CAD build for the part. Positions are in the model's coordinates, mm. Face numbers are marked on the shaded views. A direction names the side the tool comes from. Give positions to 0.01 mm unless a question says otherwise; leave off trailing zeros. Order: outer loops, then holes, each group sorted by start corner. A loop starts at its lowest first (then second) coordinate and runs counter-clockwise, first axis right, second up. Notation, with made-up numbers: (29.25, -18.75) -> (58.25, -18.75) arc R33 ccw to (58.25, 17.25) -> close; hole circle Ø8 at (-24.75, -6). An arc over 180 degrees is marked (long way). Answer as CSV lines item,"result".
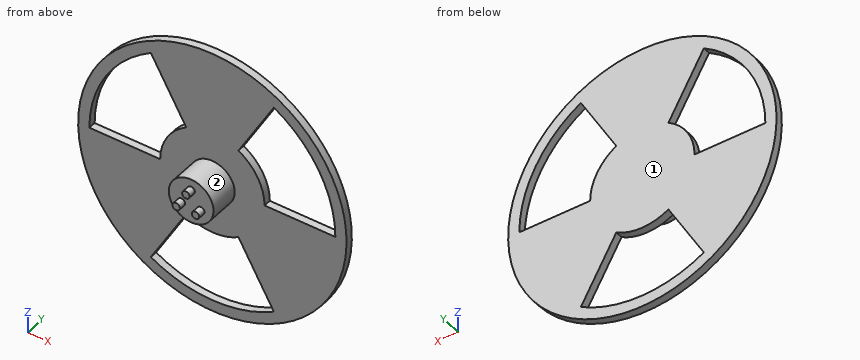
```python
from build123d import *

# Parameters (mm, degrees)
SKETCH1_R                = 18
BOSS_EXTRUDE1_DEPTH      = 1
SKETCH4_R                = 0.5
CUT_EXTRUDE2_DEPTH       = 1
BOSS_EXTRUDE2_DEPTH      = 4
BOSS_EXTRUDE2_DEPTH_BACK = 1
SKETCH5_R                = 3
BOSS_EXTRUDE3_START      = -5
SKETCH4_3_R              = 0.5
BOSS_EXTRUDE3_DEPTH      = 1


with BuildPart() as part:
    # Sketch1 → Boss-Extrude1 (new body)
    with BuildSketch(Plane(origin=(0, 0, 0), x_dir=(1, 0, 0), z_dir=(0, 1, 0))):
        with Locations(Location((0, 0, 0), (0, 0, 270))):
            Circle(SKETCH1_R)
    extrude(amount=BOSS_EXTRUDE1_DEPTH)

    # Sketch4 → Cut-Extrude2 (cut)
    with BuildSketch(Plane(origin=(0, 1, 0), x_dir=(1, 0, 0), z_dir=(0, 1, 0))):
        with Locations(Location((1.299038106, 0.75, 0), (0, 0, 270))):
            Circle(SKETCH4_R)
        with Locations(Location((0, -1.5, 0), (0, 0, 270))):
            Circle(SKETCH4_R)
        with Locations(Location((-1.299038106, 0.75, 0), (0, 0, 270))):
            Circle(SKETCH4_R)
        with BuildLine():
            Line((-3.5, 6.062177826), (-8.25, 14.289419162))
            ThreePointArc((-8.25, 14.289419162), (0, 16.5), (8.25, 14.289419162))
            Line((8.25, 14.289419162), (3.5, 6.062177826))
            ThreePointArc((3.5, 6.062177826), (0, 7), (-3.5, 6.062177826))
        make_face()
        with BuildLine():
            Line((7, 0), (16.5, 0))
            ThreePointArc((16.5, 0), (14.289419162, -8.25), (8.25, -14.289419162))
            Line((8.25, -14.289419162), (3.5, -6.062177826))
            ThreePointArc((3.5, -6.062177826), (6.062177826, -3.5), (7, 0))
        make_face()
        with BuildLine():
            Line((-3.5, -6.062177826), (-8.25, -14.289419162))
            ThreePointArc((-8.25, -14.289419162), (-14.289419162, -8.25), (-16.5, 0))
            Line((-16.5, 0), (-7, 0))
            ThreePointArc((-7, 0), (-6.062177826, -3.5), (-3.5, -6.062177826))
        make_face()
    extrude(amount=-CUT_EXTRUDE2_DEPTH, mode=Mode.SUBTRACT)

    # Sketch5 → Boss-Extrude2 (add, two sides: drawn at the far end of the back side and taken through both)
    with BuildSketch(Plane.XZ.offset(-BOSS_EXTRUDE2_DEPTH_BACK)):
        with Locations(Location((0, 0, 0), (0, 0, 270))):
            Circle(SKETCH5_R)
    extrude(amount=BOSS_EXTRUDE2_DEPTH + BOSS_EXTRUDE2_DEPTH_BACK)

    # Sketch4<3> → Boss-Extrude3 (add)
    with BuildSketch(Plane(origin=(0, 1, 0), x_dir=(1, 0, 0), z_dir=(0, 1, 0)).offset(BOSS_EXTRUDE3_START)):
        with Locations(Location((0, -1.5, 0), (0, 0, 90))):
            Circle(SKETCH4_3_R)
        with Locations(Location((-1.299038106, 0.75, 0), (0, 0, 90))):
            Circle(SKETCH4_3_R)
        with Locations(Location((1.299038106, 0.75, 0), (0, 0, 90))):
            Circle(SKETCH4_3_R)
    extrude(amount=-BOSS_EXTRUDE3_DEPTH)


solid = part.part
```
1) Band-saw the part on B-B, the plane z = 12.5. Write the cut outline in (x, y).
Data:
outline,"(-12.95, 0) -> (-10.77, 0) -> (-10.77, 1) -> (-12.95, 1) -> close; (-7.22, 0) -> (7.22, 0) -> (7.22, 1) -> (-7.22, 1) -> close; (10.77, 0) -> (12.95, 0) -> (12.95, 1) -> (10.77, 1) -> close"
2) Pin check, flat tips, straight feed: P1, Ø4, axis at x = 4, z = 9.5, coming from the -Y side; P2, Ø2, axis at x = -3.5, z = -14, coming from the -Y side; P3, Ø1.5, axis at y = -3, z = 0.5, coming from the -X side; P4, Ø3, axis at y = -1, z = 1.5, coming from the +X side. Stop position of each tip, or through.
Data:
P1,"stops at y = 0"
P2,"passes through"
P3,"stops at x = -3"
P4,"stops at x = 18"
3) Band-saw the part on D-D, the plane y = -2.9. Write the cut outline in (x, z).
Data:
outline,"circle Ø6 at (0, 0)"
4) Band-saw the part on A-A, the plane x = 0. Write the cut outline in (y, z), then the cut area to 3 significant figures.
Data:
outline,"(-5, 1) -> (-4, 1) -> (-4, -3) -> (0, -3) -> (0, -7) -> (1, -7) -> (1, 18) -> (0, 18) -> (0, 3) -> (-4, 3) -> (-4, 2) -> (-5, 2) -> close; (0, -18) -> (1, -18) -> (1, -16.5) -> (0, -16.5) -> close"
area,"51.5 mm2"
5) Wall check: line 1 along Z through (x, y) = (-6, 0.75); line 2 along Y through (x, z) = (2, -2.5); line 3 along X through (y, z) = (0.3, 10.5). Give the ranges that are in metal, low to high. Write a range as [from, to].
Data:
line 1,"z = [-16.97, -15.37], [-10.39, 3.61], [10.39, 16.97]"
line 2,"y = [0, 1]"
line 3,"x = [-14.62, -12.73], [-6.06, 6.06], [12.73, 14.62]"
6) Which spindle directions (+Z, -Z, +X, -X, +Y, -Y) get a long thin tool onto all of the face, cutting with end or side? Do the marked faces 1 and 2. Say none if no direction does.
Data:
face 1,"+Z, -Z, +X, -X, +Y"
face 2,"-Y"
7) Band-saw the part on C-C, the plane x = -11. Write the cut outline in (y, z).
Data:
outline,"(0, -14.25) -> (1, -14.25) -> (1, 0) -> (0, 0) -> close; (0, 12.3) -> (1, 12.3) -> (1, 14.25) -> (0, 14.25) -> close"
